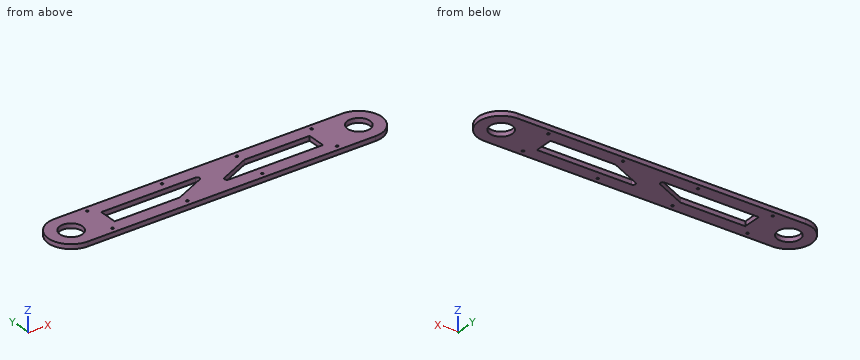
```python
from build123d import *

# Parameters (mm, degrees)
SKETCH_1_R          = 9.7
EXTRUDE_1_DEPTH     = 4
SKETCH_2_R          = 1
CUT_EXTRUDE_1_DEPTH = 10
CUT_EXTRUDE_2_DEPTH = 10


with BuildPart() as part:
    # 草图1 → 凸台-拉伸1 (new body)
    with BuildSketch(Plane.XY):
        with BuildLine():
            Line((0, 19.7), (250, 19.7))
            ThreePointArc((250, 19.7), (269.7, 0), (250, -19.7))
            Line((250, -19.7), (0, -19.7))
            ThreePointArc((0, -19.7), (-19.7, 0), (0, 19.7))
        make_face()
        Circle(SKETCH_1_R, mode=Mode.SUBTRACT)
        with Locations((250, 0)):
            Circle(SKETCH_1_R, mode=Mode.SUBTRACT)
    extrude(amount=EXTRUDE_1_DEPTH)

    # 草图2 → 切除-拉伸1 (cut)
    with BuildSketch(Plane.XY.offset(4)):
        with Locations((25, 15)):
            Circle(SKETCH_2_R)
        with Locations((90, 15)):
            Circle(SKETCH_2_R)
        with Locations((155, 15)):
            Circle(SKETCH_2_R)
        with Locations((220, 15)):
            Circle(SKETCH_2_R)
        with Locations((90, -15)):
            Circle(SKETCH_2_R)
        with Locations((155, -15)):
            Circle(SKETCH_2_R)
        with Locations((220, -15)):
            Circle(SKETCH_2_R)
        with Locations((25, -15)):
            Circle(SKETCH_2_R)
    extrude(amount=-CUT_EXTRUDE_1_DEPTH, mode=Mode.SUBTRACT)

    # 草图3 → 切除-拉伸2 (cut)
    with BuildSketch(Plane.XY.offset(4)):
        with BuildLine():
            Line((32, 8), (114.023268405, 8))
            ThreePointArc((114.023268405, 8), (115.976706085, 6.429046887), (114.86138476, 4.184081231))
            Line((114.86138476, 4.184081231), (88.462542093, -8))
            Line((88.462542093, -8), (32, -8))
            Line((32, -8), (32, 8))
        make_face()
        with BuildLine():
            Line((156.537457907, 8), (130.13861524, -4.184081231))
            ThreePointArc((130.13861524, -4.184081231), (129.023293915, -6.429046887), (130.976731595, -8))
            Line((130.976731595, -8), (213, -8))
            Line((213, -8), (213, 8))
            Line((213, 8), (156.537457907, 8))
        make_face()
    extrude(amount=-CUT_EXTRUDE_2_DEPTH, mode=Mode.SUBTRACT)


solid = part.part
```
CAD build for the part. Positions are in the model's coordinates, mm. Give positions to 0.01 mm unless a question says otherwise; leave off trailing zeros. Write each loop counter-clockwise with the first axis right and the second up, starting at its lowest first coordinate (ties: lowest second). Pieces come first, ordered by that corner, then holes. Notation, with made-up numbers: M -39.5,11 L -26.5,11 A15 cw -26.5,24 Z; hole C 44.25,87.5 d6. An arc over 180 degrees is marked long. Return JSON: item names as keys, results as strings. Group by question number.
(1) Drill centre lines: L1, parallel to Y at x = 220, z = 2.9; L2, parallel to Y at x = 163, z = 3.2; L3, parallel to X at y = 5.5, z = 1.2. Where is each one in solid material? Low to high. Write a range as [from, to].
(2) Flat gauge pins, fed straight in: pin 1 Ø1 at (y, z) = (-7, 1) entering from -X; pin 2 Ø1.2 at (x, y) = (25, 15) entering from +Z; pin 3 Ø1 at (y, z) = (4, 0.5) entering from +X. Where does each tip first touch, or does it go through?
(3) Band-saw the part on C-C (z = 2.7). State how many separate pieces and enclosed holes the cut face has, and give its area (3 significant figures).
(4) Band-saw the part on B-B (y = 0). Give the cut face in (x, z).
(5) Band-saw the part on A-A (x = 79). Give the cut face in (y, z).
Entries:
{
 "1": {"L1": "y = [-19.7, -16], [-14, 14], [16, 19.7]", "L2": "y = [-19.7, -8], [8, 19.7]", "L3": "x = [-18.92, -7.99], [7.99, 32], [115.96, 151.12], [213, 242.01], [257.99, 268.92]"},
 "2": {"pin 1": "stops at x = -18.6", "pin 2": "passes through", "pin 3": "stops at x = 269.39"},
 "3": {"separate pieces": "1", "enclosed holes": "12", "area": "8,120 mm^2"},
 "4": {"outline": "M -19.7,0 L -9.7,0 L -9.7,4 L -19.7,4 Z; M 9.7,0 L 32,0 L 32,4 L 9.7,4 Z; M 105.8,0 L 139.2,0 L 139.2,4 L 105.8,4 Z; M 213,0 L 240.3,0 L 240.3,4 L 213,4 Z; M 259.7,0 L 269.7,0 L 269.7,4 L 259.7,4 Z"},
 "5": {"outline": "M -19.7,0 L -8,0 L -8,4 L -19.7,4 Z; M 8,0 L 19.7,0 L 19.7,4 L 8,4 Z"}
}
